Read the model definition and answer for the solid it produces. Units are mm, in the model's axes. Give positions to 0.01 mm unless a question says otherwise; leave off trailing zeros. Order: outer loops, then holes, each group sorted by start corner. A loop starts at its lowest first (then second) coordinate and runs counter-clockwise, first axis right, second up.
Item 1: A cutting plane is placed at B-B (z = 21.5). Write down the section's boundary in (x, y), plus the area to 3 significant figures.
Item 2: A cutting plane is placed at D-D (x = 10). Write down the section's boundary in (y, z).
Item 3: Given pin 1 Ø6 at (y, z) = (3, 22) entering from +X; pin 2 Ø1 at (y, z) = (10.5, 1) entering from -X (3 decimals); pin 3 Ø1 at (y, z) = (9.5, 4) entering from +X; pin 4 Ø2 at (y, z) = (-3.5, 1.5) entering from +X (3 decimals), each flat-ended and moving along its own axis, determine where each tip first touches the part or whether it passes through.
Item 4: A cutting plane is placed at A-A (x = -6.5). Write down the section's boundary in (y, z), plus the area to 3 significant figures.
Item 5: A cutting plane is placed at C-C (y = 10.5). Write down the section's boundary in (x, z).
Item 6: Find the intervals of material crossed by line 1 along Z through (x, y) = (6, 13.75); line 2 along Y through (x, z) = (-3, 22.5); line 3 along Y through (x, z) = (21.5, 30), in increasing order.
from build123d import *

# Parameters (mm, degrees)
ESQUISSE1_R        = 1.75
BOSS_EXTRU_1_DEPTH = 2
BOSS_EXTRU_2_DEPTH = 30


with BuildPart() as part:
    # Esquisse1 → Boss.-Extru.1 (new body)
    with BuildSketch(Plane.XY):
        with BuildLine():
            Line((-13.285014649, -0.29563378), (-13.285014649, -5.016414934))
            ThreePointArc((-13.285014649, -5.016414934), (-12.113441773, -7.844842058), (-9.285014649, -9.016414934))
            Line((-9.285014649, -9.016414934), (2.714985351, -9.016414934))
            ThreePointArc((2.714985351, -9.016414934), (5.543412476, -7.844842058), (6.714985351, -5.016414934))
            Line((6.714985351, -5.016414934), (6.714985351, -0.348036487))
            ThreePointArc((6.714985351, -0.348036487), (21.951660894, 1.154765906), (36.998669859, 3.983585066))
            ThreePointArc((36.998669859, 3.983585066), (21.951660894, 6.812404226), (6.714985351, 8.315206619))
            Line((6.714985351, 8.315206619), (6.714985351, 12.983585066))
            ThreePointArc((6.714985351, 12.983585066), (5.543412476, 15.812012191), (2.714985351, 16.983585066))
            Line((2.714985351, 16.983585066), (-9.285014649, 16.983585066))
            ThreePointArc((-9.285014649, 16.983585066), (-12.113441773, 15.812012191), (-13.285014649, 12.983585066))
            Line((-13.285014649, 12.983585066), (-13.285014649, 8.262803913))
            ThreePointArc((-13.285014649, 8.262803913), (-28.0599618, 6.746885729), (-42.653153387, 3.983585066))
            ThreePointArc((-42.653153387, 3.983585066), (-28.0599618, 1.220284404), (-13.285014649, -0.29563378))
        make_face()
        with Locations((-9.285014649, 12.983585066)):
            Circle(ESQUISSE1_R, mode=Mode.SUBTRACT)
        with Locations((-9.285014649, -5.016414934)):
            Circle(ESQUISSE1_R, mode=Mode.SUBTRACT)
        with Locations((2.714985351, -5.016414934)):
            Circle(ESQUISSE1_R, mode=Mode.SUBTRACT)
        with Locations((2.714985351, 12.983585066)):
            Circle(ESQUISSE1_R, mode=Mode.SUBTRACT)
    extrude(amount=BOSS_EXTRU_1_DEPTH)

    # Esquisse2 → Boss.-Extru.2 (add)
    with BuildSketch(Plane.XY.offset(2)):
        with BuildLine():
            ThreePointArc((36.998669859, 3.983585066), (-2.827241764, 8.575554846), (-42.653153387, 3.983585066))
            ThreePointArc((-42.653153387, 3.983585066), (-2.827241764, -0.608384714), (36.998669859, 3.983585066))
        make_face()
    extrude(amount=BOSS_EXTRU_2_DEPTH)


solid = part.part
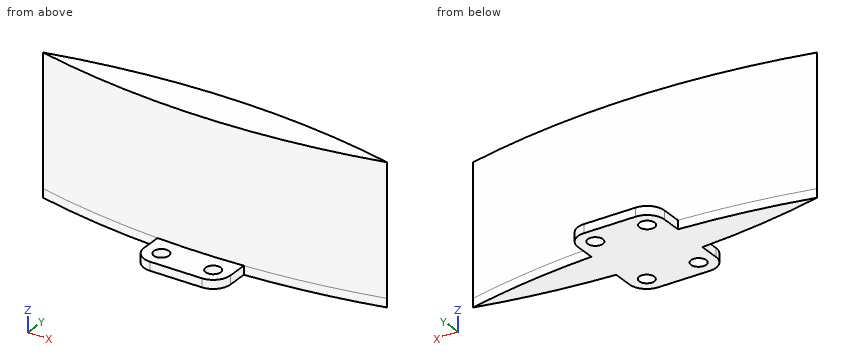
Response values:
1. outline: (-42.65, 3.98) arc R175 ccw to (37, 3.98) arc R175 ccw to start
1. area: 489 mm2
2. outline: (-0.14, 0) - (8.1, 0) - (8.1, 32) - (-0.14, 32) - close
3. pin 1: stops at x = 37
3. pin 2: stops at x = -13.285
3. pin 3: passes through
3. pin 4: stops at x = 6.715
4. outline: (-9.02, 0) - (16.98, 0) - (16.98, 2) - (8.54, 2) - (8.54, 32) - (-0.57, 32) - (-0.57, 2) - (-9.02, 2) - close
4. area: 325 mm2
5. outline: (-13.29, 0) - (6.71, 0) - (6.71, 2) - (-13.29, 2) - close
6. line 1: z = 0 to 2
6. line 2: y = -0.61 to 8.58
6. line 3: y = 1.09 to 6.88
